Design review of the part built by this model. Coordinates are the model's own, in mm. A direction names the side the tool comes from. Give positions to 0.01 mm unless a question says otherwise; leave off trailing zeros. Loops run counter-clockwise (first coordinate to the right, second up) from the corner with the lowest first, then second, coordinate; pieces in that order, holes last. Notation, with made-up numbers: M 32,-6.5 L 39,-6.5 A14 cw 39,-0.5 Z; hole C 18.5,64 d8. An arc over 180 degrees is marked long. Answer as CSV lines item,"result".
```python
from build123d import *

# Parameters (mm, degrees)
SKETCH1_W           = 12.04
SKETCH1_H           = 7.58
SKETCH1_W_2         = 8.04
SKETCH1_H_2         = 3.58
BOSS_EXTRUDE1_DEPTH = 8
SKETCH1_2_W         = 12.04
SKETCH1_2_H         = 7.58
SKETCH1_2_W_2       = 8.04
SKETCH1_2_H_2       = 3.58
BOSS_EXTRUDE2_DEPTH = 2
EXTRUDE_THIN1_START = -12.04
EXTRUDE_THIN1_DEPTH = 12.04
SKETCH5_W           = 12.04
SKETCH5_H           = 7.58
SKETCH5_W_2         = 8.04
SKETCH5_H_2         = 3.58
BOSS_EXTRUDE4_DEPTH = 10
SKETCH5_4_W         = 12.04
SKETCH5_4_H         = 7.58
BOSS_EXTRUDE5_DEPTH = 2
CHAMFER1_SIZE       = 1.5


with BuildPart() as part:
    # Sketch1 → Boss-Extrude1 (new body)
    with BuildSketch(Plane.XY):
        Rectangle(SKETCH1_W, SKETCH1_H)
        Rectangle(SKETCH1_W_2, SKETCH1_H_2, mode=Mode.SUBTRACT)
    extrude(amount=BOSS_EXTRUDE1_DEPTH)

    # Sketch1<2> → Boss-Extrude2 (add)
    # profile 1 of 2: a face of its own
    with BuildSketch(Plane.XY):
        Rectangle(SKETCH1_2_W, SKETCH1_2_H)
        Rectangle(SKETCH1_2_W_2, SKETCH1_2_H_2, mode=Mode.SUBTRACT)
    # profile 2 of 2: a face of its own
    with BuildSketch(Plane.XY):
        Rectangle(SKETCH1_2_W_2, SKETCH1_2_H_2)
    extrude(amount=-BOSS_EXTRUDE2_DEPTH)

    # Sketch3 → Extrude-Thin1 (add)
    with BuildSketch(Plane(origin=(6.02, 9.81, 0), x_dir=(0, -1, 0), z_dir=(1, 0, 0)).offset(EXTRUDE_THIN1_START)):
        with BuildLine():
            Line((13.6, 2), (9.52, 2))
            ThreePointArc((9.52, 2), (9.350894106, 9.75), (8.843898328, 17.485247384))
            Line((8.843898328, 17.485247384), (12.908372696, 17.840842814))
            Line((12.908372696, 17.840842814), (12.734061211, 19.83323221))
            Line((12.734061211, 19.83323221), (6.665855308, 19.302332986))
            ThreePointArc((6.665855308, 19.302332986), (7.352797663, 9.662761226), (7.508614841, 0))
            Line((7.508614841, 0), (13.6, 0))
            Line((13.6, 0), (13.6, 2))
        make_face()
    extrude(amount=EXTRUDE_THIN1_DEPTH)

    # Sketch5 → Boss-Extrude4 (add)
    with BuildSketch(Plane(origin=(0, -2.22544681, -17.764471695), x_dir=(-1, 0, 0), z_dir=(0, 0.08715574274765182, -0.9961946980917462))):
        with Locations((0, 2.913739678)):
            Rectangle(SKETCH5_W, SKETCH5_H)
        with Locations((0, 2.913739678)):
            Rectangle(SKETCH5_W_2, SKETCH5_H_2, mode=Mode.SUBTRACT)
    extrude(amount=BOSS_EXTRUDE4_DEPTH)

    # Sketch5<4> → Boss-Extrude5 (add)
    with BuildSketch(Plane(origin=(0, -2.22544681, -17.764471695), x_dir=(-1, 0, 0), z_dir=(0, 0.08715574274765182, -0.9961946980917462))):
        with Locations((0, 2.913739678)):
            Rectangle(SKETCH5_4_W, SKETCH5_4_H)
    extrude(amount=BOSS_EXTRUDE5_DEPTH)

    # Chamfer1
    chamfer1_edges = [part.edges().sort_by_distance(p)[0] for p in [
        (0, -3.79, -2),
        (0, 3.79, -2),
        (-6.02, -2.662593983, -22.821816304),
        (6.02, -2.662593983, -22.821816304),
        (0, -3.098372696, -17.840842814),
        (6.02, -3.79, 3),
        (-6.02, -3.79, 3),
        (-6.02, 3.79, 3),
        (6.02, 3.79, 3),
        (0, 4.452783115, -17.180202284),
        (6.02, 4.888561829, -22.161175774),
        (-6.02, 4.888561829, -22.161175774),
    ]]
    chamfer(chamfer1_edges, length=CHAMFER1_SIZE - 0.0001)  # a hair under: the kernel refuses the full size


solid = part.part
```
1. To check wall thickness, follow L1, parallel to X at y = -1.75, z = 6; L2, parallel to Y at x = 4.5, z = 6.5; L3, parallel to Y at x = -2.5, z = -23.5. State the ranges of each line that lie inside material, in increasing order. Write a range as [from, to].
Answer block:
L1,"[-6.02, -4.02], [4.02, 6.02]"
L2,"[-3.79, 3.79]"
L3,"[-2.6, -0.6], [3, 5.01]"
2. For faces 5 (the flat face through (0, -1, -2)), 6 (the flat face through (0.06, 2.98, -23.28)), 7 (the flat face through (4.02, 0, 4)), 8 (the flat face through (-5.26, 3.05, 3.07)), 9 (the cylindrical face through (-0.08, 2.46, -9.77)), list the 3-axis set-ups (+Z, -Z, +X, -X, +Y, -Y) from which the entire face can be reached by the end or side of a thin tool; tool diameter is ignored.
Answer block:
face 5,"+X, -X, -Y"
face 6,"-Z"
face 7,"+Z"
face 8,"+Z, -X, +Y"
face 9,"+X, -X, +Y"
3. For P1, Ø4.5, axis at x = 0.5, z = 5, coming from the +Y side; P2, Ø1.5, axis at y = 2.5, z = 4, coming from the -X side; P3, Ø4, axis at x = 4, z = -12, coming from the -Y side; P4, Ø1.5, axis at y = -2.5, z = -18.5, coming from the -X side, all flat-tipped, find the tip position at first contact; note any pin that passes through.
Answer block:
P1,"y = 3.79"
P2,"x = -6.02"
P3,"y = 0.47"
P4,"x = -5.81"
4. The part is to be moulded in two halves that separate along Y. For faces 1 (the flat face through (6.02, 1, -10)), 2 (the flat face through (-0.08, 3.03, -1.26)), 3 (the flat face through (-0.056, 0.827, -19.505)), 4 (the flat face through (0, 0, 0)), say which applies: pulls with the +Y half, pulls with the -Y half, needs draft (parallel to the pull), parting line crosses it, or undercut.
Answer block:
face 1,"needs draft"
face 2,"pulls with the +Y half"
face 3,"undercut"
face 4,"undercut"
5. We need section A-A, the plane z = 1. Write out the cut boundary in (x, y).
Answer block:
outline,"M -6.02,-2.29 L -4.52,-3.79 L 4.52,-3.79 L 6.02,-2.29 L 6.02,2.29 L 4.52,3.79 L -4.52,3.79 L -6.02,2.29 Z; hole M -4.02,-1.79 L 4.02,-1.79 L 4.02,1.79 L -4.02,1.79 Z"
6. We need section C-C, the plane z = -19. Write out the cut boundary in (x, y).
Answer block:
outline,"M -6.02,-1.49 L -4.83,-2.69 L 4.83,-2.69 L 6.02,-1.49 L 6.02,3.11 L 4.52,4.61 L -4.52,4.61 L -6.02,3.11 Z"
